Autodesk Inventor part; units mm, degrees
ref_plane "YZ Plane" through (0, 0, 0) normal (1, 0, 0) x (0, 1, 0)
ref_plane "XZ Plane" through (0, 0, 0) normal (0, 1, 0) x (-1, 0, 0)
ref_plane "XY Plane" through (0, 0, 0) normal (0, 0, 1) x (1, 0, 0)
sketch "Sketch1" plane through (0, 0, 0) normal (0, 0, 1) x (1, 0, 0)
  line L0 (0, 0) -> (40, 0)
  line L1 (40, 0) -> (40, 15)
  line L2 (40, 15) -> (0, 15)
  line L3 (0, 15) -> (0, 0)
  dimension "d0" = 40
  dimension "d1" = 15
extrude "Extrusion1" add sketch "Sketch1" along normal blind 5
sketch "Sketch2" plane through (0, 15, 0) normal (0, 1, 0) x (1, 0, 0)
  line L0 (35, -5) -> (5, -5)
  line L1 (5, -5) -> (5, -20)
  line L2 (5, -20) -> (35, -20)
  line L3 (28, -16.75) -> (12, -16.75)
  line L4 (12, -16.75) -> (12, -8.25)
  line L5 (12, -8.25) -> (28, -8.25)
  circle A0 centre (30, -12.5) radius 1.5
  circle A1 centre (10, -12.5) radius 1.5
  line L6 (28, -16.75) -> (28, -8.25)
  line L7 (0, 0) -> (0, -5)
  line L8 (40, -5) -> (0, -5)
  line L9 (35, -5) -> (35, -20)
  dimension "d4" = 8.5
  dimension "d7" = 4.25
  dimension "d8" = 4.25
  dimension "d9" = 3
  dimension "d10" = 3
  dimension "d11" = 20
  dimension "d13" = 16
  dimension "d14" = 2
  dimension "d28" = 5
  dimension "d29" = 5
  dimension "d30" = 5
  dimension "d31" = 15
  dimension "d32" = 3.25
extrude "Extrusion2" add sketch "Sketch2" against normal blind 3
sketch "Sketch3" plane through (0, 0, 5) normal (0, 0, 1) x (1, 0, 0)
  circle A0 centre (35, 5) radius 2.2
  circle A1 centre (5, 5) radius 2.2
  line L0 (40, 0) -> (40, 15)
  line L1 (0, 15) -> (0, 0)
  line L2 (0, 0) -> (40, 0)
  point P0 (40, 17)
  point P1 (0, 17)
  dimension "d17" = 4.4
  dimension "d18" = 5
  dimension "d19" = 5
  dimension "d20" = 4.4
  dimension "d21" = 5
  dimension "d22" = 5
extrude "Extrusion3" cut sketch "Sketch3" against normal blind 10
chamfer "Chamfer1" distance 5 angle 45 2 edges at (5, 13.5, 20) (35, 13.5, 20)
properties part number "xt60_plug_mount_v2"
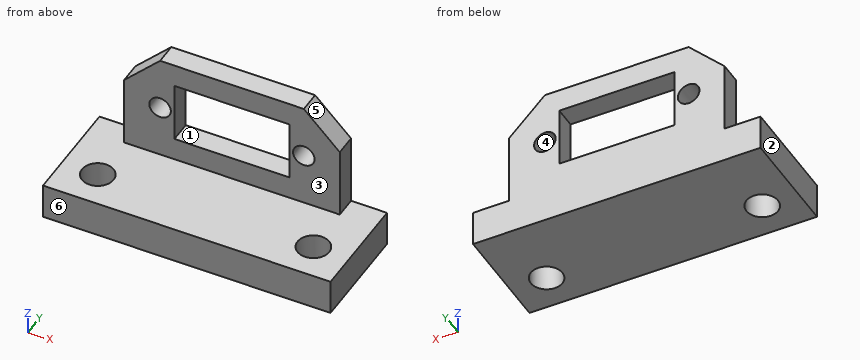
Read the model definition and answer for the solid it produces. Units are mm, in the model's axes. Face numbers are marked on the shaded views. A direction names the side the tool comes from. Give positions to 0.01 mm unless a question says otherwise; leave off trailing zeros. Write each loop counter-clockwise with the first axis right and the second up, starting at its lowest first coordinate (ties: lowest second). Pieces come first, ordered by that corner, then holes. Notation, with made-up numbers: (33, 45) -> (40, 45) arc R16 ccw to (40, 74) -> close; hole circle Ø1 at (17.25, 73). An arc over 180 degrees is marked (long way). Answer as a JSON object with one key per item and string values. Group by question number.
1) Find section A-A (x = 13). Write down the section's boundary in (y, z), and give its area (3 significant figures).
2) Find section D-D (x = 32). Write down the section's boundary in (y, z).
3) A tool of negligible diameter and unlimited length cuts with its end or side. For the marked faces 1, 2 and 3, from which of +Z, -Z, +X, -X, +Y, -Y can it reach the whole face along a straight path? Write none if from no direction.
4) Each of these flat-tipped pins is pushed along its axis until it touches: P1, Ø1.5, axis at y = 13.5, z = 9, coming from the +X side; P2, Ø1.5, axis at x = 11.5, y = 6.5, coming from the +Z side; P3, Ø1.5, axis at y = 14, z = 11.5, coming from the -X side. Where does it stop, or does it pass through?
5) Find section B-B (z = 12.5). Write down the section's boundary in (x, y), and give its area (3 significant figures).
6) Consider L1, parallel to X at y = 13.8, z = 12.5; L2, parallel to Y at x = 5, z = 1.6; L3, parallel to Z at x = 30, y = 13.65. Determine where each line is inside the solid, lowest interval first. Write a range as from..to.
7) The mould has two halves that part along Z. Classify the marked faces 4, 5 and 6: +Z half, -Z half, draft (parallel to the pull), parting line (faces both ways), or undercut.
8) Find section C-C (y = 5). Write down the section's boundary in (x, z).
Values follow:
{
 "1": {"outline": "(0, 0) -> (15, 0) -> (15, 8.25) -> (12, 8.25) -> (12, 5) -> (0, 5) -> close; (12, 16.75) -> (15, 16.75) -> (15, 20) -> (12, 20) -> close", "area": "94.5 mm2"},
 "2": {"outline": "(0, 0) -> (15, 0) -> (15, 18) -> (12, 18) -> (12, 5) -> (0, 5) -> close"},
 "3": {"face 1": "+Y, -Y", "face 2": "+Z, -Z, -X, +Y, -Y", "face 3": "+Z, +X, -X, -Y"},
 "4": {"P1": "stops at x = 35", "P2": "stops at z = 5", "P3": "stops at x = 5"},
 "5": {"outline": "(5, 12) -> (8.5, 12) -> (8.5, 15) -> (5, 15) -> close; (11.5, 12) -> (12, 12) -> (12, 15) -> (11.5, 15) -> close; (28, 12) -> (28.5, 12) -> (28.5, 15) -> (28, 15) -> close; (31.5, 12) -> (35, 12) -> (35, 15) -> (31.5, 15) -> close", "area": "24.0 mm2"},
 "6": {"L1": "x = 5..8.5, 11.5..12, 28..28.5, 31.5..35", "L2": "y = 0..2.8, 7.2..15", "L3": "z = 0..11, 14..20"},
 "7": {"face 4": "undercut", "face 5": "+Z half", "face 6": "draft"},
 "8": {"outline": "(0, 0) -> (2.8, 0) -> (2.8, 5) -> (0, 5) -> close; (7.2, 0) -> (32.8, 0) -> (32.8, 5) -> (7.2, 5) -> close; (37.2, 0) -> (40, 0) -> (40, 5) -> (37.2, 5) -> close"}
}
